Model file for the job. Use its own axes, mm. Face numbers are marked on the shaded views. Coordinates: 2 decimals unless noted, no trailing zeros. Loops run counter-clockwise (first coordinate to the right, second up) from the corner with the lowest first, then second, coordinate; pieces in that order, holes last.
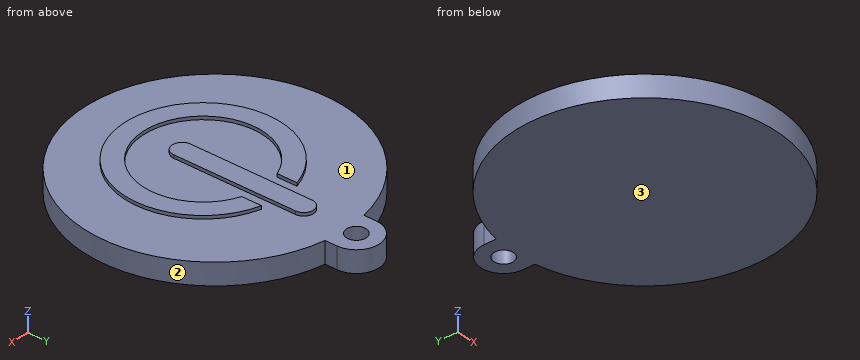
from build123d import *

# Parameters (mm, degrees)
EXTRUDE_DEPTH = 3.3
SKETCH001_R   = 1.5
POCKET_DEPTH  = 3.301
PAD_DEPTH     = 0.5


with BuildPart() as part:
    # Sketch → Extrude (new body)
    with BuildSketch(Plane.XY):
        with BuildLine():
            ThreePointArc((3.5, 21.5), (0, 25), (-3.5, 21.5))
            Line((-3.5, 21.5), (-3.5, 19.691369))
            ThreePointArc((-3.5, 19.691369), (0, -20), (3.5, 19.691369))
            Line((3.5, 19.691369), (3.5, 21.5))
        make_face()
    extrude(amount=EXTRUDE_DEPTH)

    # Sketch001 → Pocket (cut, through all)
    with BuildSketch(Plane.XY.offset(3.3)):
        with Locations((0, 21.5)):
            Circle(SKETCH001_R)
    extrude(amount=-POCKET_DEPTH, mode=Mode.SUBTRACT)

    # Sketch002 → Pad (new body)
    with BuildSketch(Plane.XY.offset(3.3)):
        with BuildLine():
            Line((-1.5, 13.5), (-1.5, -5))
            ThreePointArc((-1.5, -5), (0, -6.5), (1.5, -5))
            Line((1.5, 13.5), (1.5, -5))
            ThreePointArc((1.5, 13.5), (0, 15), (-1.5, 13.5))
        make_face()
        with BuildLine():
            ThreePointArc((-3.2, 9.765466), (0, -13.8), (3.2, 9.765466))
            Line((3.2, 9.765466), (3.2, 6.765466))
            ThreePointArc((-3.2, 6.765466), (0, -10.943698), (3.2, 6.765466))
            Line((-3.2, 9.765466), (-3.2, 6.765466))
        make_face()
    extrude(amount=PAD_DEPTH)


solid = part.part
Q1. Drill centre lines: line 1 (X direction, y = -1.8, z = 3.65); line 2 (Y direction, x = 0, z = 1.85); line 3 (Z direction, x = -5.5, y = -6). Where is each one in solid material? Low to high.
Answers:
line 1: x = -12 to -9.14, -1.5 to 1.5, 9.14 to 12
line 2: y = -20 to 20, 23 to 25
line 3: z = 0 to 3.3
Q2. Flat gauge pins, fed straight in: P1, Ø0.6, axis at y = 5, z = 3.5, coming from the +X side; P2, Ø0.6, axis at y = 1.5, z = 3.5, coming from the -X side; P3, Ø1.4, axis at y = 20.5, z = 1.5, coming from the -X side; P4, Ø1.8, axis at x = 0, y = 21.5, coming from the -Z side. Where does each tip first touch, or does it go through?
Answers:
P1: stops at x = 19.42
P2: stops at x = -19.96
P3: stops at x = -3.5
P4: passes through
Q3. Slice it at D-D (y = -1.5). List the corners of the cut face in (x, z).
Answers:
outline: (-19.94, 0) - (19.94, 0) - (19.94, 3.3) - (12, 3.3) - (12, 3.8) - (9.14, 3.8) - (9.14, 3.3) - (1.5, 3.3) - (1.5, 3.8) - (-1.5, 3.8) - (-1.5, 3.3) - (-9.14, 3.3) - (-9.14, 3.8) - (-12, 3.8) - (-12, 3.3) - (-19.94, 3.3) - close
Q4. Slice it at B-B (z = 2.8). List the corners of the cut face in (x, y), and give its area (3 significant figures).
Answers:
outline: (-3.5, 19.69) arc R20 ccw (long way) to (3.5, 19.69) - (3.5, 21.5) arc R3.5 ccw to (-3.5, 21.5) - close; hole circle Ø3 at (0, 21.5)
area: 1,280 mm2
Q5. Slice it at A-A (x = 0). List the corners of the cut face in (y, z).
Answers:
outline: (-20, 0) - (20, 0) - (20, 3.3) - (15, 3.3) - (15, 3.8) - (-6.5, 3.8) - (-6.5, 3.3) - (-10.94, 3.3) - (-10.94, 3.8) - (-13.8, 3.8) - (-13.8, 3.3) - (-20, 3.3) - close; (23, 0) - (25, 0) - (25, 3.3) - (23, 3.3) - close
Q6. Slice it at C-C (y = 21). List the corners of the cut face in (x, z), and give its area (3 significant figures).
Answers:
outline: (-3.5, 0) - (-1.41, 0) - (-1.41, 3.3) - (-3.5, 3.3) - close; (1.41, 0) - (3.5, 0) - (3.5, 3.3) - (1.41, 3.3) - close
area: 13.8 mm2
Q7. Mould opens along X. For the marked faces 1, 2 and 3 say: +X half, -X half, draft (parallel to the pull), parting line (faces both ways), or undercut.
Answers:
face 1: undercut
face 2: parting line
face 3: draft
